The listing builds one solid part. Answer for the finished solid, in the listing's coordinates (mm). Face numbers are marked on the shaded views. A direction names the side the tool comes from. Give positions to 0.01 mm unless a question says otherwise; leave off trailing zeros. Answer as CSV lines item,"result". Start each with the question number.
1. Section A-A on x = -28 is taken. Count the separate pieces of the cut face and the enclosed holes in it, and give its area (3 significant figures).
2. Which of the six approach directions +Z, -Z, +X, -X, +Y, -Y give full straight-line access (tool end or side, diameter ignored) to the marked faces 1, 2, 3 and 4?
3. Flat-ended cylindrical pins translate along their axes: pin 1 (1 mm diameter, centred on x = 35, z = 18, fed in from -Y); pin 2 (1.5 mm diameter, centred on y = -38, z = 22.5, fed in from -X); pin 3 (2 mm diameter, centred on x = 37, z = 27, fed in from -Y). Find the tip coordinate at first contact, or state that the pin passes through.
4. Consider line 1 along X through (y, z) = (-26, 13); line 2 along Y through (x, z) = (-20.5, 9); line 3 along X through (y, z) = (45, 48). Determine where each line is inside the solid, lowest interval first. Write a range as [from, to].
5. Determine the mould class of the marked faces 5, 6 and 7 for opening direction Y: +Y half, -Y half, draft (parallel to the pull), parting line (faces both ways), or undercut.
from build123d import *

# Parameters (mm, degrees)
ESQUISSE1_R                   = 50
BOSS_EXTRU_1_DEPTH            = 50
ENL_V_MAT_EXTRU_1_DEPTH       = 9.999999999999984
R_P_TITION_CIRCULAIRE1_COUNT  = 4
CHANFREIN1_SIZE               = 5
ESQUISSE11_R                  = 13.500000000000002
BOSS_EXTRU_3_DEPTH            = 4.999999999999999
ESQUISSE4_R                   = 37.50000000000001
ENL_V_MAT_EXTRU_2_DEPTH       = 50
CHANFREIN2_SIZE               = 5
BOSS_EXTRU_2_DEPTH            = 4.9999999999999964
ESQUISSE5_R                   = 1.7500000000000004
ENL_V_MAT_EXTRU_3_DEPTH       = 5
ESQUISSE7_R                   = 2.000000000000003
ENL_V_MAT_EXTRU_4_DEPTH       = 5.999999999999993
R_P_TITION_CIRCULAIRE2_COUNT  = 4
CHANFREIN3_SIZE               = 2
ESQUISSE8_W                   = 13
ESQUISSE8_H                   = 19.000000000000004
ESQUISSE8_W_2                 = 12.999999999999996
ESQUISSE8_H_2                 = 18.999999999999993
ENL_V_MAT_EXTRU_5_DEPTH       = 18.999999999999986
ENL_V_MAT_EXTRU_6_REACH       = 106.174
ENL_V_MAT_EXTRU_8_DEPTH       = 19.000000000000004
BOSS_EXTRU_4_DEPTH            = 45.000000000000014
ENL_V_START                   = 17
ESQUISSE12_R                  = 13.500000000000002
ENL_V_MAT_EXTRU_10_DEPTH      = 17
ESQUISSE15_R                  = 3.0000000000000013
ENL_V_MAT_EXTRU_11_DEPTH      = 17
ESQUISSE16_R                  = 11.99999999999999
ENL_V_MAT_EXTRU_12_DEPTH      = 0.9999999999999931
CHANFREIN4_SIZE               = 7
CHANFREIN5_SIZE               = 2
ENL_V_MAT_EXTRU_13_DEPTH      = 5.999999999999993
ENL_V_MAT_EXTRU_14_DEPTH      = 0.9999999999999931
ENL_V_MAT_EXTRU_14_DEPTH_BACK = 5.999999999999993
ESQUISSE19_R                  = 0.9999999999999983
ENL_V_MAT_EXTRU_15_DEPTH      = 5.999999999999993
ESQUISSE20_R                  = 6.499999999999999
ENL_V_MAT_EXTRU_16_DEPTH      = 13
ENL_V_MAT_EXTRU_17_DEPTH      = 7.9999999999999964
ENL_V_MAT_EXTRU_17_DEPTH_BACK = 7.9999999999999964
ESQUISSE21_R                  = 11.500000000000004


with BuildPart() as part:
    # Esquisse1 → Boss.-Extru.1 (new body)
    with BuildSketch(Plane.XY):
        Circle(ESQUISSE1_R)
    extrude(amount=BOSS_EXTRU_1_DEPTH)

    # Esquisse3 → Enlèv. mat.-Extru.1 (cut)
    with BuildSketch(Plane(origin=(0, 50, 0), x_dir=(1, 0, 0), z_dir=(0, 1, 0))):
        Polygon((0, -45), (0, -4.9999999999999964), (-45.00000000000001, -5.000000000000003), (-45.00000000000001, -45.00000000000001), align=None)
        Polygon((44.99999999999999, -4.99999999999999), (0, -4.9999999999999964), (0, -45), (45, -44.99999999999999), align=None)
    enl_v_mat_extru_1 = extrude(amount=-ENL_V_MAT_EXTRU_1_DEPTH, mode=Mode.SUBTRACT)

    # Répétition circulaire1: Enlèv. mat.-Extru.1 ×4 about axis
    r_p_tition_circulaire1_axis = Axis((0, 0, 0), (0, 0, 1))
    for i in range(1, R_P_TITION_CIRCULAIRE1_COUNT):
        add(enl_v_mat_extru_1.rotate(r_p_tition_circulaire1_axis, i * 360 / R_P_TITION_CIRCULAIRE1_COUNT), mode=Mode.SUBTRACT)

    # Chanfrein1
    chanfrein1_edges = [part.edges().sort_by_distance(p)[0] for p in [
        (0, 40.000000000000014, 45),
        (40.000000000000014, -8.88e-15, 45),
        (40.000000000000014, -8.88e-15, 4.9999999999999964),
        (-4.9e-15, -40.000000000000014, 4.9999999999999964),
        (-40.000000000000014, 4.44e-15, 4.9999999999999964),
        (-4.9e-15, -40.000000000000014, 45),
        (-40.000000000000014, 4.44e-15, 45),
        (0, 40.000000000000014, 4.9999999999999964),
    ]]
    chamfer(chanfrein1_edges, length=CHANFREIN1_SIZE)

    # Esquisse11 → Boss.-Extru.3 (add)
    with BuildSketch(Plane(origin=(-2.499999999999722, 2.657e-14, -2.49999999999975), x_dir=(-0.7071067811865515, -7.515584591766378e-15, 0.7071067811865436), z_dir=(-0.7071067811865436, 7.515584591766462e-15, -0.7071067811865515))):
        with Locations((53.67514421272203, -2.4659e-13)):
            Circle(ESQUISSE11_R)
    extrude(amount=-BOSS_EXTRU_3_DEPTH)

    # Esquisse4 → Enlèv. mat.-Extru.2 (cut)
    with BuildSketch(Plane(origin=(0, 0, 0), x_dir=(-1, 0, 0), z_dir=(0, 0, -1))):
        Circle(ESQUISSE4_R)
    extrude(amount=-ENL_V_MAT_EXTRU_2_DEPTH, mode=Mode.SUBTRACT)

    # Chanfrein2
    chanfrein2_edges = [part.edges().sort_by_distance(p)[0] for p in [
        (37.50000000000001, 4.59e-15, 50),
    ]]
    chamfer(chanfrein2_edges, length=CHANFREIN2_SIZE)

    # Esquisse6 → Boss.-Extru.2 (add)
    with BuildSketch(Plane(origin=(0, 0, 0), x_dir=(-1, 0, 0), z_dir=(0, 0, -1))):
        with BuildLine():
            ThreePointArc((34.369317712168815, 15.000000000000002), (2.3e-15, 37.500000000000014), (-34.369317712168815, 15.000000000000004))
            Line((-34.36931771216881, 15), (34.36931771216881, 15))
        make_face()
        with BuildLine():
            Line((34.36931771216881, -15), (-34.36931771216881, -15))
            ThreePointArc((-34.369317712168815, -14.999999999999996), (-6.89e-15, -37.500000000000014), (34.369317712168815, -15.000000000000009))
        make_face()
    extrude(amount=-BOSS_EXTRU_2_DEPTH)

    # Esquisse5 → Enlèv. mat.-Extru.3 (cut)
    with BuildSketch(Plane(origin=(0, 0, 0), x_dir=(-1, 0, 0), z_dir=(0, 0, -1))):
        with Locations((-20.875, 20.844288786139956)):
            Circle(ESQUISSE5_R)
        with Locations((20.875, 20.844288786139956)):
            Circle(ESQUISSE5_R)
        with Locations((-20.875, -20.844288786139956)):
            Circle(ESQUISSE5_R)
        with Locations((20.875, -20.844288786139956)):
            Circle(ESQUISSE5_R)
    extrude(amount=-ENL_V_MAT_EXTRU_3_DEPTH, mode=Mode.SUBTRACT)

    # Esquisse7 → Enlèv. mat.-Extru.4 (cut)
    with BuildSketch(Plane.XY.offset(50)):
        with Locations((-45, 0)):
            Circle(ESQUISSE7_R)
    enl_v_mat_extru_4 = extrude(amount=-ENL_V_MAT_EXTRU_4_DEPTH, mode=Mode.SUBTRACT)

    # Répétition circulaire2: Enlèv. mat.-Extru.4 ×4 about axis
    r_p_tition_circulaire2_axis = Axis((0, 7.856e-14, 0), (0, 0, 1))
    for i in range(1, R_P_TITION_CIRCULAIRE2_COUNT):
        add(enl_v_mat_extru_4.rotate(r_p_tition_circulaire2_axis, i * 360 / R_P_TITION_CIRCULAIRE2_COUNT), mode=Mode.SUBTRACT)

    # Chanfrein3
    chanfrein3_edges = [part.edges().sort_by_distance(p)[0] for p in [
        (0, 37.50000000000002, 4.9999999999999964),
        (5.33e-15, -37.50000000000001, 4.9999999999999964),
    ]]
    chamfer(chanfrein3_edges, length=CHANFREIN3_SIZE)

    # Esquisse8 → Enlèv. mat.-Extru.5 (cut)
    with BuildSketch(Plane.XZ.offset(40.00000000000002)):
        with Locations((-19.999999999999975, 25.000000000000014)):
            Rectangle(ESQUISSE8_W, ESQUISSE8_H)
        Polygon((6.500000000000003, 15.500000000000291), (6.500000000000003, 34.500000000000284), (-6.499999999999999, 34.500000000000284), (-6.499999999999996, 15.500000000000291), align=None)
        with Locations((19.99999999999998, 25.00000000000001)):
            Rectangle(ESQUISSE8_W_2, ESQUISSE8_H_2)
    extrude(amount=-ENL_V_MAT_EXTRU_5_DEPTH, mode=Mode.SUBTRACT)

    # Enlèv. mat.-Extru.6: up to this face of the body (flat: up to its plane)
    enl_v_mat_extru_6_end = Plane(part.part.faces().sort_by_distance((-26.5, -33.266499161, 25))[0])
    # Esquisse9 → Enlèv. mat.-Extru.6 (cut, up to the picked face)
    with BuildSketch(Plane.ZY.offset(-26.49999999999998), mode=Mode.PRIVATE) as enl_v_mat_extru_6_sk1:
        Polygon((15.500000000000014, -26.53299832284323), (15.500000000000014, -37.00000000000002), (34.50000000000001, -37.00000000000002), (34.50000000000001, -26.532998322843227), align=None)
    enl_v_mat_extru_6_tool1 = split(extrude(enl_v_mat_extru_6_sk1.sketch, amount=ENL_V_MAT_EXTRU_6_REACH, mode=Mode.PRIVATE), bisect_by=enl_v_mat_extru_6_end, keep=Keep.BOTH, mode=Mode.PRIVATE)
    add(enl_v_mat_extru_6_tool1.solids().sort_by(Axis((26.5, -31.766499, 25), (-1, 0, 0)))[0], mode=Mode.SUBTRACT)

    # Esquisse10 → Enlèv. mat.-Extru.8 (cut)
    with BuildSketch(Plane(origin=(0, -37.00000000000002, 0), x_dir=(1, 0, 0), z_dir=(0, 1, 0))):
        Polygon((30.49999999999998, -38.50000000000001), (30.49999999999997, -11.500000000000014), (-30.499999999999968, -11.500000000000014), (-30.499999999999968, -38.500000000000014), align=None)
    extrude(amount=ENL_V_MAT_EXTRU_8_DEPTH, mode=Mode.SUBTRACT)

    # Esquisse14 → Boss.-Extru.4 (add)
    with BuildSketch(Plane(origin=(0, 0, 0), x_dir=(-1, 0, 0), z_dir=(0, 0, -1))):
        with BuildLine():
            ThreePointArc((34.36931771216881, 15), (19.369317712168808, 1.84e-15), (34.36931771216881, -15))
            ThreePointArc((34.36931771216881, -15), (37.50000000000001, 0), (34.36931771216881, 15))
        make_face()
    extrude(amount=-BOSS_EXTRU_4_DEPTH)

    # Esquisse12 → Enlèv. mat.-Extru.10 (cut)
    with BuildSketch(Plane(origin=(-2.4999999999997247, 2.657e-14, -2.499999999999752), x_dir=(-0.7071067811865515, -7.515584591766378e-15, 0.7071067811865436), z_dir=(-0.7071067811865436, 7.515584591766462e-15, -0.7071067811865515)).offset(ENL_V_START)):
        with Locations((53.67514421272203, -2.4659e-13)):
            Circle(ESQUISSE12_R)
    extrude(amount=-ENL_V_MAT_EXTRU_10_DEPTH, mode=Mode.SUBTRACT)

    # Esquisse15 → Enlèv. mat.-Extru.11 (cut)
    with BuildSketch(Plane(origin=(-2.4999999999997247, 2.657e-14, -2.499999999999752), x_dir=(-0.7071067811865515, -7.515584591766378e-15, 0.7071067811865436), z_dir=(-0.7071067811865436, 7.515584591766462e-15, -0.7071067811865515))):
        with Locations((53.67514421272203, -2.4659e-13)):
            Circle(ESQUISSE15_R)
    extrude(amount=-ENL_V_MAT_EXTRU_11_DEPTH, mode=Mode.SUBTRACT)

    # Esquisse16 → Enlèv. mat.-Extru.12 (cut)
    with BuildSketch(Plane(origin=(-2.4999999999997247, 2.657e-14, -2.499999999999752), x_dir=(-0.7071067811865515, -7.515584591766378e-15, 0.7071067811865436), z_dir=(-0.7071067811865436, 7.515584591766462e-15, -0.7071067811865515))):
        with Locations((53.67514421272203, -2.4659e-13)):
            Circle(ESQUISSE16_R)
    extrude(amount=-ENL_V_MAT_EXTRU_12_DEPTH, mode=Mode.SUBTRACT)

    # Chanfrein4
    chanfrein4_edges = [part.edges().sort_by_distance(p)[0] for p in [
        (37.50000000000001, 4.59e-15, 0),
    ]]
    chamfer(chanfrein4_edges, length=CHANFREIN4_SIZE)

    # Chanfrein5
    chanfrein5_edges = [part.edges().sort_by_distance(p)[0] for p in [
        (-50, 6.12e-15, 0),
    ]]
    chamfer(chanfrein5_edges, length=CHANFREIN5_SIZE)

    # Esquisse17 → Enlèv. mat.-Extru.13 (cut)
    with BuildSketch(Plane(origin=(40.00000000000002, -1.3966e-13, 0), x_dir=(0, 0, -1), z_dir=(1, -3.49e-15, 0))):
        Polygon((-15.000000000000014, -13.999999999999998), (-35.000000000000014, -14), (-35.000000000000014, 13.999999999999998), (-15.000000000000014, 14.000000000000002), align=None)
    extrude(amount=-ENL_V_MAT_EXTRU_13_DEPTH, mode=Mode.SUBTRACT)

    # Esquisse18 → Enlèv. mat.-Extru.14 (cut, two sides: drawn at the far end of the back side and taken through both)
    with BuildSketch(Plane(origin=(34.7886475735979, -1.4656e-13, -2.414e-14), x_dir=(-6.9e-16, 0, -1), z_dir=(1, -4.21e-15, -6.9e-16)).offset(-ENL_V_MAT_EXTRU_14_DEPTH_BACK)):
        Polygon((-10.00000000000004, -18.999999999999968), (-10.00000000000004, 19.000000000000032), (-40.00000000000004, 19.00000000000003), (-40.00000000000004, -18.99999999999997), align=None)
    extrude(amount=ENL_V_MAT_EXTRU_14_DEPTH + ENL_V_MAT_EXTRU_14_DEPTH_BACK, mode=Mode.SUBTRACT)

    # Esquisse19 → Enlèv. mat.-Extru.15 (cut)
    with BuildSketch(Plane(origin=(40.00000000000002, -1.3966e-13, 0), x_dir=(0, 0, -1), z_dir=(1, -3.49e-15, 0))):
        with Locations(Location((-36.500000000000014, -13.000000000000002, 0), (0, 0, 90))):
            Circle(ESQUISSE19_R)
        with Locations(Location((-13.500000000000005, -13.000000000000002, 0), (0, 0, 90))):
            Circle(ESQUISSE19_R)
    enl_v_mat_extru_15 = extrude(amount=-ENL_V_MAT_EXTRU_15_DEPTH, mode=Mode.SUBTRACT)

    # Symétrie1: Enlèv. mat.-Extru.15 across plane
    add(enl_v_mat_extru_15.mirror(Plane.ZX), mode=Mode.SUBTRACT)

    # Esquisse20 → Enlèv. mat.-Extru.16 (cut)
    with BuildSketch(Plane(origin=(0, 40.00000000000002, 0), x_dir=(1, 0, 0), z_dir=(0, 1, 0))):
        with Locations(Location((-14.999999999999986, -25.00000000000001, 0), (0, 0, 270))):
            Circle(ESQUISSE20_R)
    extrude(amount=-ENL_V_MAT_EXTRU_16_DEPTH, mode=Mode.SUBTRACT)

    # Esquisse21 → Enlèv. mat.-Extru.17 (cut, two sides: drawn at the far end of the back side and taken through both)
    with BuildSketch(Plane(origin=(0, 29.00000000000002, 0), x_dir=(1, 0, 0), z_dir=(0, 1, 0)).offset(-ENL_V_MAT_EXTRU_17_DEPTH_BACK)):
        with Locations((-14.999999999999986, -25.00000000000001)):
            Circle(ESQUISSE21_R)
    extrude(amount=ENL_V_MAT_EXTRU_17_DEPTH + ENL_V_MAT_EXTRU_17_DEPTH_BACK, mode=Mode.SUBTRACT)


solid = part.part
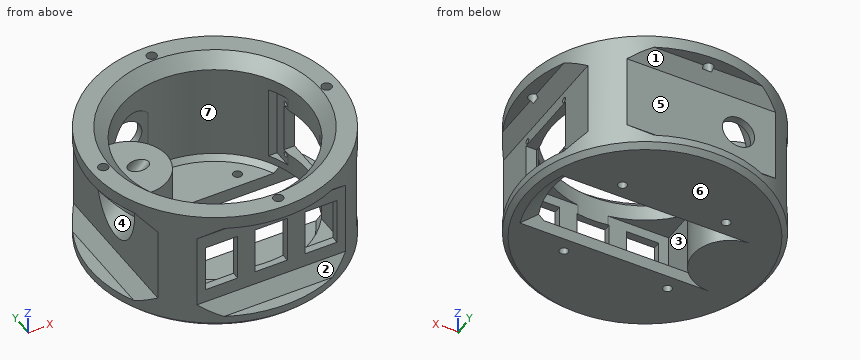
Checks:
1,separate pieces,"3"
1,enclosed holes,"0"
1,area,"2,520 mm²"
2,face 1,"+X, -X, +Y"
2,face 2,"+X, -X, -Y"
2,face 3,"none"
2,face 4,"-X"
3,pin 1,"stops at y = -36.19"
3,pin 2,"stops at x = -33.35"
3,pin 3,"stops at y = -34.7"
4,line 1,"x = [-40, -30.5], [30.5, 40]"
4,line 2,"y = [-41, -31.4], [-5.71, 5.71], [31.4, 41]"
4,line 3,"x = [-21.79, -2], [2, 21.79]"
5,face 5,"+Y half"
5,face 6,"draft"
5,face 7,"undercut"
